Model file for the job. Use its own axes, mm. Round coordinates to 2 decimals unless told otherwise and drop trailing zeros. Loops run counter-clockwise (first coordinate to the right, second up) from the corner with the lowest first, then second, coordinate; pieces in that order, holes last. Notation, with made-up numbers: (69, 83.5) -> (78, 83.5) arc R32 ccw to (78, 121.5) -> close; hole circle Ø9 at (87, 15). An arc over 180 degrees is marked (long way). Use a Markdown table: item, result.
from build123d import *

# Parameters (mm, degrees)
SKETCH1_R           = 76.2
BOSS_EXTRUDE1_DEPTH = 6.35


with BuildPart() as part:
    # Sketch1 → Boss-Extrude1 (new body)
    with BuildSketch(Plane(origin=(0, 0, 0), x_dir=(1, 0, 0), z_dir=(0, 1, 0))):
        Polygon((0, 0), (0, -25.4), (-304.8, -25.4), (-304.8, 0), (-330.2, 0), (-330.2, 304.8), (-304.8, 304.8), (-304.8, 330.2), (0, 330.2), (0, 304.8), (25.4, 304.8), (25.4, 0), align=None)
        with Locations((-152.4, 152.4)):
            Circle(SKETCH1_R, mode=Mode.SUBTRACT)
    extrude(amount=BOSS_EXTRUDE1_DEPTH)


solid = part.part
Q1. Band-saw the part on C-C, the plane x = -152.4. Give the cut face in (y, z), plus the area to 3 significant figures.
Results list:
| item | result |
|---|---|
| outline | (0, -330.2) -> (6.35, -330.2) -> (6.35, -228.6) -> (0, -228.6) -> close; (0, -76.2) -> (6.35, -76.2) -> (6.35, 25.4) -> (0, 25.4) -> close |
| area | 1,290 mm² |
Q2. Pull direction Y, two halves, no side cores. Call faces 1 (the face through (-168.919, 3.131, -78.012)), 2 (the face through (-229, 0, -155)), 3 (the face through (-229, 6.35, -155)): released by +Y, released by -Y, zero draft, split by the parting line, or undercut.
Results list:
| item | result |
|---|---|
| face 1 | zero draft |
| face 2 | released by -Y |
| face 3 | released by +Y |
Q3. Band-saw the part on A-A, the plane y = 4.5. Give the cut face in (x, z), plus the area to 3 significant figures.
Results list:
| item | result |
|---|---|
| outline | (-330.2, -304.8) -> (-304.8, -304.8) -> (-304.8, -330.2) -> (0, -330.2) -> (0, -304.8) -> (25.4, -304.8) -> (25.4, 0) -> (0, 0) -> (0, 25.4) -> (-304.8, 25.4) -> (-304.8, 0) -> (-330.2, 0) -> close; hole circle Ø152.4 at (-152.4, -152.4) |
| area | 106,000 mm² |
Q4. Band-saw the part on B-B, the plane z = -152.4. Give the cut face in (x, y), plus the area to 3 significant figures.
Results list:
| item | result |
|---|---|
| outline | (-330.2, 0) -> (-228.6, 0) -> (-228.6, 6.35) -> (-330.2, 6.35) -> close; (-76.2, 0) -> (25.4, 0) -> (25.4, 6.35) -> (-76.2, 6.35) -> close |
| area | 1,290 mm² |
Q5. Drill centre lines: L1, parallel to X at y = 2.75, z = -152.4; L2, parallel to X at y = 3, z = -114. Where is each one in solid material? Low to high. Write a range as from..to.
Results list:
| item | result |
|---|---|
| L1 | x = -330.2..-228.6, -76.2..25.4 |
| L2 | x = -330.2..-218.22, -86.58..25.4 |
Q6. Flat gauge pins, fed straight in: pin 1 (1.9 mm diameter, centred on x = -313.5, y = 3.5, fed in from -Z); pin 2 (3 mm diameter, centred on x = -27, z = -142.5, fed in from -Y); pin 3 (1.9 mm diameter, centred on y = 2, z = -311.5, fed in from +X); pin 4 (3 mm diameter, centred on y = 4, z = 12, fed in from -X). Where does each tip first touch, or does it go through?
Results list:
| item | result |
|---|---|
| pin 1 | stops at z = -304.8 |
| pin 2 | stops at y = 0 |
| pin 3 | stops at x = 0 |
| pin 4 | stops at x = -304.8 |
